from build123d import *

# Parameters (mm, degrees)
F0_R     = 4
F1_DEPTH = 3.5


with BuildPart() as f1:
    # F0 (on Front) → F1 (new body)
    with BuildSketch(Plane.XZ):
        with BuildLine():
            Line((0, -2), (0, 0))
            Line((0, 0), (-84, 0))
            Line((-84, 0), (-87.3775810443, -3.6867256867))
            Line((-87.3775810443, -3.6867256867), (-86.2715633383, -4.7))
            Line((-86.2715633383, -4.7), (-86.2715633383, -11))
            Line((-86.2715633383, -11), (-80.7715633383, -11))
            Line((-80.7715633383, -11), (-54.5028455385, -14.493488966))
            Line((-54.5028455385, -14.493488966), (-25, -40))
            Line((-25, -40), (-20.3, -40))
            Line((-20.3, -40), (-21.7744337692, -34.4973382611))
            ThreePointArc((-21.7744337692, -34.4973382611), (-21.6018612832, -33.629757787), (-20.8085079429, -33.238519216))
            Line((-20.8085079429, -33.238519216), (-2.1117333157, -33.238519216))
            ThreePointArc((-2.1117333157, -33.238519216), (1.5298666074, -31.7301191391), (3.0382666843, -28.088519216))
            ThreePointArc((3.0382666843, -28.088519216), (2.3691920714, -25.5500536017), (0.5358171017, -23.6711696954))
            Line((0.5358171017, -23.6711696954), (-2.1348951645, -22.0868976918))
            ThreePointArc((-2.1348951645, -22.0868976918), (-2.3213319674, -21.9801363334), (-2.5044046725, -21.8677038925))
            ThreePointArc((-2.5044046725, -21.8677038925), (-5.3568950896, -13.6469284918), (2, -9))
            Line((2, -9), (5, -9))
            ThreePointArc((5, -9), (7.8284271247, -7.8284271247), (9, -5))
            Line((9, -5), (9, -2))
            Line((9, -2), (0, -2))
        make_face()
        with Locations((-20, -25)):
            Circle(F0_R, mode=Mode.SUBTRACT)
        with BuildLine():
            Line((-2.1348951645, -22.0868976918), (-2.5044046725, -21.8677038925))
            ThreePointArc((-2.5044046725, -21.8677038925), (-2.3213319674, -21.9801363334), (-2.1348951645, -22.0868976918))
        make_face()
    extrude(amount=F1_DEPTH)


solid = f1.part
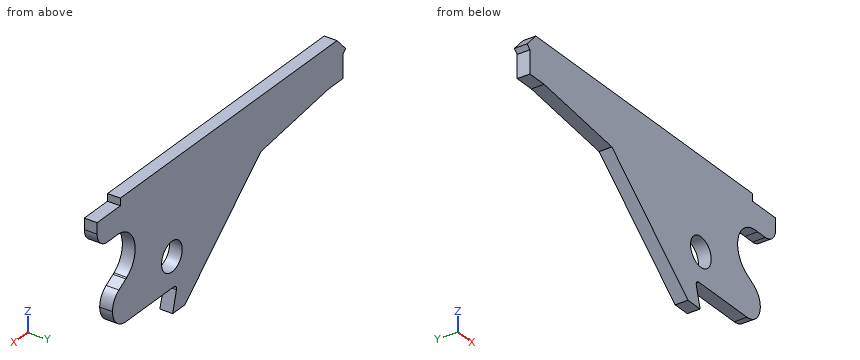
Here's how the part is built. I have some questions about the finished solid (model axes, mm). Give positions to 0.01 mm unless a question says otherwise; leave off trailing zeros. Loops run counter-clockwise (first coordinate to the right, second up) from the corner with the lowest first, then second, coordinate; pieces in that order, holes last. Notation, with made-up numbers: (13, -1.75) -> (35, -1.75) arc R24 ccw to (35, 15.25) -> close; hole circle Ø9 at (32.5, 87). An arc over 180 degrees is marked (long way). Answer as a JSON object with one key per item and string values. Group by question number.
Item 1: I need wall thicknesses on L1, parallel to Z at x = -20, y = -1.1; L2, parallel to Z at x = -54.5, y = -3.25; L3, parallel to X at y = -0.6, z = -23.5. Which ranges of each line are inside material? Lowest first, please.
Item 2: Imagine slicing it at A-A on y = -1.3. Write out the boundary of the cut face in (x, z), then the cut area to 3 significant figures.
Item 3: Imagine slicing it at B-B on x = -17. Write out the boundary of the cut face in (y, z).
Item 4: Will these pins go through, and if not, where does the flat tip stop? pin 1 (1 mm diameter, centred on y = -1, z = -7.5, fed in from -X); pin 2 (1 mm diameter, centred on x = -82, y = -2.5, fed in from -Z); pin 3 (1.6 mm diameter, centred on y = -1.5, z = -1, fed in from +X).
Item 5: Imagine slicing it at C-C on z = -27. Write out the boundary of the cut face in (x, y).
Item 6: Imagine slicing it at D-D on z = -16. Write out the boundary of the cut face in (x, y), then the cut area to 3 significant figures.
Answer list:
{
 "1": {"L1": "z = -33.24 to -29, -21 to 0", "L2": "z = -14.5 to 0", "L3": "x = -44.09 to -23.71, -16.29 to 0.25"},
 "2": {"outline": "(-87.38, -3.69) -> (-86.27, -4.7) -> (-86.27, -11) -> (-80.77, -11) -> (-54.5, -14.49) -> (-25, -40) -> (-20.3, -40) -> (-21.77, -34.5) arc R1 cw to (-20.81, -33.24) -> (-2.11, -33.24) arc R5.15 ccw to (0.54, -23.67) -> (-2.5, -21.87) arc R7 cw to (2, -9) -> (5, -9) arc R4 ccw to (9, -5) -> (9, -2) -> (0, -2) -> (0, 0) -> (-84, 0) -> close; hole circle Ø8 at (-20, -25)", "area": "2,020 mm2"},
 "3": {"outline": "(-3.5, -33.24) -> (0, -33.24) -> (0, -27.65) -> (-3.5, -27.65) -> close; (-3.5, -22.35) -> (0, -22.35) -> (0, 0) -> (-3.5, 0) -> close"},
 "4": {"pin 1": "stops at x = -86.27", "pin 2": "stops at z = -11", "pin 3": "stops at x = 0"},
 "5": {"outline": "(-40.04, -3.5) -> (-23.46, -3.5) -> (-23.46, 0) -> (-40.04, 0) -> close; (-16.54, -3.5) -> (2.92, -3.5) -> (2.92, 0) -> (-16.54, 0) -> close"},
 "6": {"outline": "(-52.76, -3.5) -> (-5.75, -3.5) -> (-5.75, 0) -> (-52.76, 0) -> close", "area": "165 mm2"}
}
